```python
from build123d import *

# Parameters (mm, degrees)
F0_W      = 30
F0_H      = 30
F1_DEPTH  = 3
F2_W      = 30
F2_H      = 3
F3_DEPTH  = 57
F4_R      = 2.375
F5_DEPTH  = 3
F6_R      = 1.5
F7_DEPTH  = 3
F10_DEPTH = 30


with BuildPart() as f1:
    # F0 (on Top) → F1 (new body)
    with BuildSketch(Plane.XY):
        Rectangle(F0_W, F0_H)
    extrude(amount=F1_DEPTH)

    # F2 (on face) → F3 (join)
    with BuildSketch(Plane.XY.offset(3)):
        with Locations((0, 13.5)):
            Rectangle(F2_W, F2_H)
    extrude(amount=F3_DEPTH)

    # F4 (on face) → F5 (cut, through all)
    with BuildSketch(Plane.XY.offset(3)):
        with Locations((0, -1.3210215056)):
            Circle(F4_R)
    extrude(amount=-F5_DEPTH, mode=Mode.SUBTRACT)

    # F6 (on face) → F7 (cut, through all)
    with BuildSketch(Plane.XZ.offset(-12)):
        with Locations((-6.75, 44)):
            Circle(F6_R)
        with BuildLine():
            ThreePointArc((8.25, 44), (6.75, 45.5), (5.25, 44))
            ThreePointArc((5.25, 44), (6.75, 42.5), (8.25, 44))
        make_face()
    extrude(amount=-F7_DEPTH, mode=Mode.SUBTRACT)

    # F9 (on offset) → F10 (join, through all)
    with BuildSketch(Plane(origin=(-15, 0, 0), x_dir=(0, -1, 0), z_dir=(-1, 0, 0))):
        Polygon((-12, 5.1583419554), (-9.9405581132, 3), (-6.9405581132, 3), (-12, 8.1583419554), align=None)
    extrude(amount=-F10_DEPTH)


solid = f1.part
```
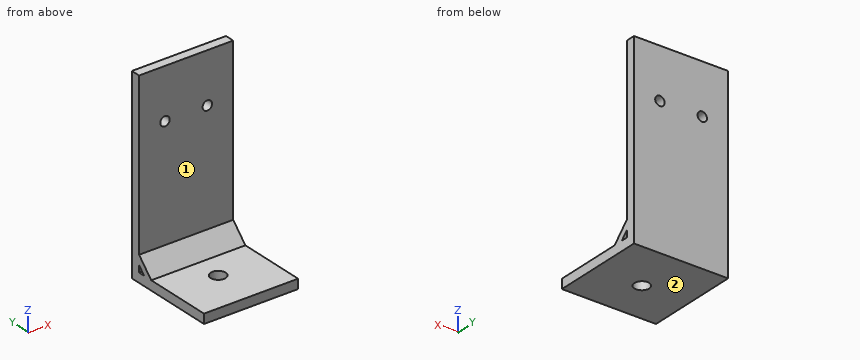
Geometry check sheet. Reference: the model listing, model coordinates, mm. Face numbers are marked on the shaded views. A direction names the side the tool comes from. Coordinates: 2 decimals unless noted, no trailing zeros. Order: outer loops, then holes, each group sorted by start corner. A loop starts at its lowest first (then second) coordinate and runs counter-clockwise, first axis right, second up. Notation, with made-up numbers: (17.25, 22) - (44.25, 22) arc R11 ccw to (44.25, 28) - close; hole circle Ø8 at (-32, -34.75). An arc over 180 degrees is marked (long way). Answer as a JSON object with one key per item and string values. Group by question number.
Item 1: Sectioned sample at B-B, the plane z = 44. Record the cut outline in (x, y).
Item 2: Sectioned sample at D-D, the plane y = 11.25. Record the cut outline in (x, z), and give its area (3 significant figures).
Item 3: Sectioned sample at C-C, the plane x = -10.75. Record the cut outline in (y, z), and give its area (3 significant figures).
Item 4: Depth check by flat-ended pin: pin 1 Ø10 at (x, y) = (-2.5, -4.5) entering from +Z; pin 2 Ø1.7 at (x, z) = (-2, 4) entering from -Y; pin 3 Ø10 at (x, y) = (11.5, 5) entering from +Z. Enter the tip coordinate at first touch or a pass-through.
Item 5: Scan lines: probe 1 along Y at (x, z) = (0, 1.3); probe 2 along Z at (x, y) = (6.75, 13.7); probe 3 along Z at (x, y) = (-7.25, -7). Record each from-to range of solid material in increasing order.
Item 6: Sectioned sample at A-A, the plane x = 0. Record the cut outline in (y, z).
Item 7: Tool access check on the marked faces 1 and 2. Record the directions out of +Z, -Z, +X, -X, +Y, -Y that give a thin tool (end or side, any length) a straight path to the whole face; none if there is none.
Resolved:
{
 "1": {"outline": "(-15, 12) - (-8.25, 12) - (-8.25, 15) - (-15, 15) - close; (-5.25, 12) - (5.25, 12) - (5.25, 15) - (-5.25, 15) - close; (8.25, 12) - (15, 12) - (15, 15) - (8.25, 15) - close"},
 "2": {"outline": "(-15, 0) - (15, 0) - (15, 3) - (-15, 3) - close; (-15, 4.37) - (15, 4.37) - (15, 7.39) - (-15, 7.39) - close", "area": "181 mm^2"},
 "3": {"outline": "(-15, 0) - (15, 0) - (15, 60) - (12, 60) - (12, 8.16) - (6.94, 3) - (-15, 3) - close; hole (9.94, 3) - (12, 3) - (12, 5.16) - close", "area": "272 mm^2"},
 "4": {"pin 1": "z = 3", "pin 2": "y = 7.09", "pin 3": "z = 6.12"},
 "5": {"probe 1": "-15 to -3.7, 1.05 to 15", "probe 2": "0 to 42.5, 45.5 to 60", "probe 3": "0 to 3"},
 "6": {"outline": "(-15, 0) - (-3.7, 0) - (-3.7, 3) - (-15, 3) - close; (1.05, 0) - (15, 0) - (15, 60) - (12, 60) - (12, 8.16) - (6.94, 3) - (1.05, 3) - close; hole (9.94, 3) - (12, 3) - (12, 5.16) - close"},
 "7": {"face 1": "+Z, +X, -X, -Y", "face 2": "-Z, +X, -X, +Y, -Y"}
}
